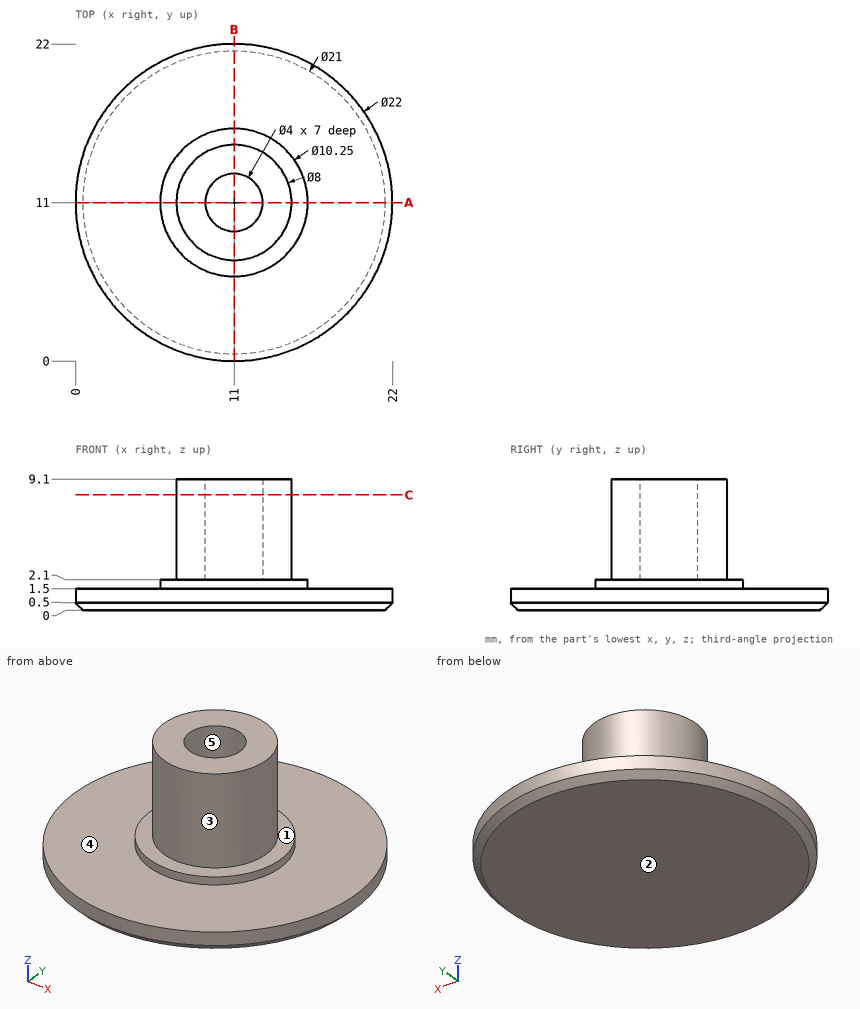
Job drawing, mm, ordinate dimensions from the low corner. One solid piece. A direction names the side the tool comes from. Give positions to 0.01 mm unless a question says otherwise; leave off trailing zeros. Order: outer loops, then holes, each group sorted by start corner. A loop starts at its lowest first (then second) coordinate and runs counter-clockwise, first axis right, second up. Notation, with made-up numbers: (45, 32.5) - (86, 32.5) arc R26 cw to (86, 63.5) - close; hole circle Ø1 at (36, 77). An arc over 180 degrees is marked (long way). Return JSON: item names as keys, results as strings.
1) Cut at C-C, the plane z = 8. Give the cut face in (x, y), plus the area to 3 significant figures.
Geometry says:
{"outline": "circle Ø8 at (11, 11); hole circle Ø4 at (11, 11)", "area": "37.7 mm²"}
2) Cut at A-A, the plane y = 11. Give the cut face in (x, z) (3 decimals), plus the area to 3 significant figures.
Geometry says:
{"outline": "(0, 0.5) - (0.5, 0) - (21.5, 0) - (22, 0.5) - (22, 1.5) - (16.125, 1.5) - (16.125, 2.1) - (15, 2.1) - (15, 9.1) - (13, 9.1) - (13, 2.1) - (9, 2.1) - (9, 9.1) - (7, 9.1) - (7, 2.1) - (5.875, 2.1) - (5.875, 1.5) - (0, 1.5) - close", "area": "66.9 mm²"}
3) 3-axis set-ups, long thin cutter, end or side, ignore diameter. For the marked faces 1 and 2: which of +Z, -Z, +X, -X, +Y, -Y reach the whole face in a straight line?
Geometry says:
{"face 1": "+Z", "face 2": "-Z, +X, -X, +Y, -Y"}
4) Pull direction X, two halves, no side cores. Call the marked faces 3, 4 and 5: pulls with the +X half, pulls with the -X half, needs draft (parallel to the pull), parting line crosses it, or undercut.
Geometry says:
{"face 3": "parting line crosses it", "face 4": "needs draft", "face 5": "undercut"}
5) Probe line 1 (Y direction, x = 11, z = 5.25); line 2 (Z direction, x = 6.5, y = 4); line 3 (Z direction, x = 9.5, y = 10). List the from-to ranges inside material, lowest first. Write a range as from..to.
Geometry says:
{"line 1": "7..9, 13..15", "line 2": "0..1.5", "line 3": "0..2.1"}
6) Flat gauge pins, fed straight in: P1, Ø1, axis at y = 5.5, z = 1, coming from the -X side; P2, Ø5, axis at x = 15, z = 2.5, coming from the +Y side; P3, Ø3, axis at x = 11, y = 11, coming from the +Z side. Where does each tip first touch, or does it go through?
Geometry says:
{"P1": "x = 1.2", "P2": "y = 21.87", "P3": "z = 2.1"}
